Source: three-view drawing plus pictorial views. Frame: mm from the lowest corner of the part. Round coordinates to 2 decimals unless told otherwise and drop trailing zeros. Write each loop counter-clockwise with the first axis right and the second up, starting at its lowest first coordinate (ties: lowest second). Pieces come first, ordered by that corner, then holes. Notation, with made-up numbers: (68.5, 48.25) -> (89.5, 48.25) arc R18 cw to (89.5, 66.25) -> close; hole circle Ø5 at (48, 4). An arc over 180 degrees is marked (long way). Put each result on its own line as item: value.
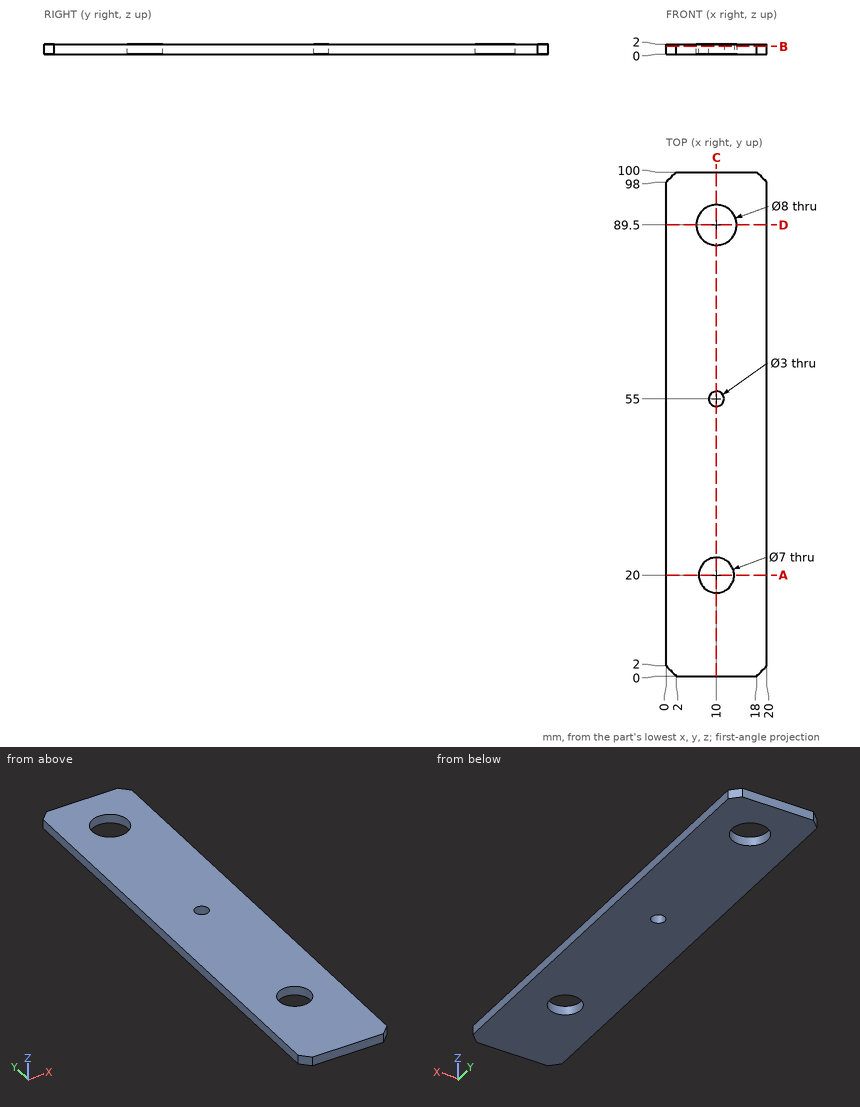
Q1. Cut plane C-C on x = 10. Output: boundary loops of the cut face in (y, z).
Ans:
outline: (0, 0) -> (16.5, 0) -> (16.5, 2) -> (0, 2) -> close; (23.5, 0) -> (53.5, 0) -> (53.5, 2) -> (23.5, 2) -> close; (56.5, 0) -> (85.5, 0) -> (85.5, 2) -> (56.5, 2) -> close; (93.5, 0) -> (100, 0) -> (100, 2) -> (93.5, 2) -> close
Q2. Cut plane A-A on y = 20. Output: boundary loops of the cut face in (x, z), and give its area (3 significant figures).
Ans:
outline: (0, 0) -> (6.5, 0) -> (6.5, 2) -> (0, 2) -> close; (13.5, 0) -> (20, 0) -> (20, 2) -> (13.5, 2) -> close
area: 26.0 mm^2
Q3. Cut plane D-D on y = 89.5. Output: boundary loops of the cut face in (x, z), and give its area (3 significant figures).
Ans:
outline: (0, 0) -> (6, 0) -> (6, 2) -> (0, 2) -> close; (14, 0) -> (20, 0) -> (20, 2) -> (14, 2) -> close
area: 24.0 mm^2
Q4. Material intervals for line 1 (Y direction, x = 10, z = 1.4); line 2 (Y direction, x = 12.75, z = 0.1); line 3 (Y direction, x = 8.75, z = 1.45), sorted ascending. Write a range as [from, to].
Ans:
line 1: y = [0, 16.5], [23.5, 53.5], [56.5, 85.5], [93.5, 100]
line 2: y = [0, 17.83], [22.17, 86.6], [92.4, 100]
line 3: y = [0, 16.73], [23.27, 54.17], [55.83, 85.7], [93.3, 100]
Q5. Cut plane B-B on z = 1.55. Output: boundary loops of the cut face in (x, y), and give its area (3 significant figures).
Ans:
outline: (0, 2) -> (2, 0) -> (18, 0) -> (20, 2) -> (20, 98) -> (18, 100) -> (2, 100) -> (0, 98) -> close; hole circle Ø8 at (10, 89.5); hole circle Ø7 at (10, 20); hole circle Ø3 at (10, 55)
area: 1,900 mm^2
